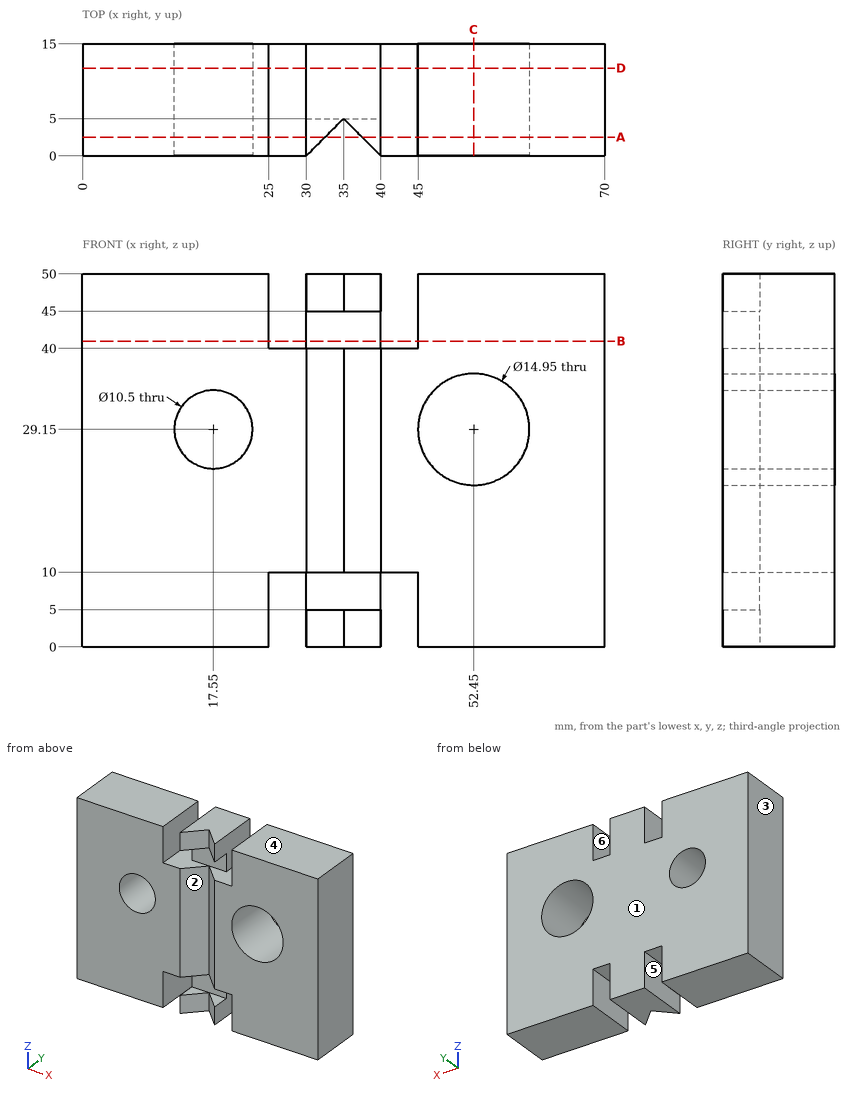
Part print with two shaded views. Sizes in mm from the minimum x, y, z corner. A direction names the side the tool comes from. Round coordinates to 2 decimals unless told otherwise and drop trailing zeros. Loops run counter-clockwise (first coordinate to the right, second up) from the corner with the lowest first, then second, coordinate; pieces in that order, holes last. Notation, with made-up numbers: M 25.25,-6.75 L 43.25,-6.75 A25 cw 43.25,27.25 Z; hole C 26,-30 d10. An arc over 180 degrees is marked long. Return JSON: item names as keys, results as strings. Group by question number.
(1) Drop flat-ended pins along their axis: P1, Ø1.5, axis at x = 33.5, y = 2, coming from the -Z side; P2, Ø5, axis at x = 41.5, y = 6.5, coming from the +Z side; P3, Ø5.5, axis at x = 35.5, z = 8.5, coming from the -Y side; P4, Ø1.5, axis at x = 35.5, z = 42, coming from the -Y side. Give the stop position or say it passes through.
(2) Wall check: probe 1 along X at (y, z) = (5.5, 7); probe 2 along Z at (x, y) = (17.55, 7.25); probe 3 along Z at (x, y) = (52.45, 4.75) (3 decimals). Give the ranges that are in metal, low to high. Write a range as [from, to].
(3) Mould opens along X. For the marked faces 1, 2 and 3 say: +X half, -X half, draft (parallel to the pull), parting line (faces both ways), or undercut.
(4) Saw through at D-D, the plane y = 11.75. List the corners of the cut face in (x, z) (3 decimals), and give its area (3 significant figures).
(5) Tool access for the marked faces 4, 5 and 6: list every direction of +Z, -Z, +X, -X, +Y, -Y with a clear straight run to the whole face (end or side of a thin tool).
(6) Saw through at B-B, the plane z = 41. List the corners of the cut face in (x, y).
(7) Saw through at A-A, the plane y = 2.5. Give the number of separate pieces and of enclosed holes in the cut face, and give its area (3 significant figures).
(8) Saw through at C-C, the plane x = 52.45. List the corners of the cut face in (y, z) (3 decimals), and give its area (3 significant figures).
Answer list:
{
 "1": {"P1": "through", "P2": "z = 50", "P3": "y = 2.2", "P4": "y = 5"},
 "2": {"probe 1": "[0, 25], [30, 40], [45, 70]", "probe 2": "[0, 23.9], [34.4, 50]", "probe 3": "[0, 21.675], [36.625, 50]"},
 "3": {"face 1": "draft", "face 2": "undercut", "face 3": "-X half"},
 "4": {"outline": "M 0,0 L 25,0 L 25,10 L 30,10 L 30,0 L 40,0 L 40,10 L 45,10 L 45,0 L 70,0 L 70,50 L 45,50 L 45,40 L 40,40 L 40,50 L 30,50 L 30,40 L 25,40 L 25,50 L 0,50 Z; hole C 17.55,29.15 d10.5; hole C 52.45,29.15 d14.95", "area": "3,040 mm2"},
 "5": {"face 4": "+Z, +X, -X, +Y, -Y", "face 5": "-Z, +Y, -Y", "face 6": "+Z, +Y, -Y"},
 "6": {"outline": "M 0,0 L 25,0 L 25,15 L 0,15 Z; M 30,5 L 40,5 L 40,15 L 30,15 Z; M 45,0 L 70,0 L 70,15 L 45,15 Z"},
 "7": {"separate pieces": "6", "enclosed holes": "2", "area": "2,740 mm2"},
 "8": {"outline": "M 0,0 L 15,0 L 15,21.675 L 0,21.675 Z; M 0,36.625 L 15,36.625 L 15,50 L 0,50 Z", "area": "526 mm2"}
}
